Can you work these out from the drawing? Everything is in mm from the part's minimum corner. A direction names the side the tool comes from. Give positions to 0.01 mm unless a question says otherwise; leave off trailing zeros. Loops run counter-clockwise (first coordinate to the right, second up) from the corner with the lowest first, then second, coordinate; pieces in that order, holes last. Notation, with made-up numbers: (42.5, 42.5) - (98.5, 42.5) arc R23 cw to (98.5, 63.5) - close; hole circle Ø8 at (-34, -19). An arc over 180 degrees is marked (long way). Answer in a Markdown table with one row per item.
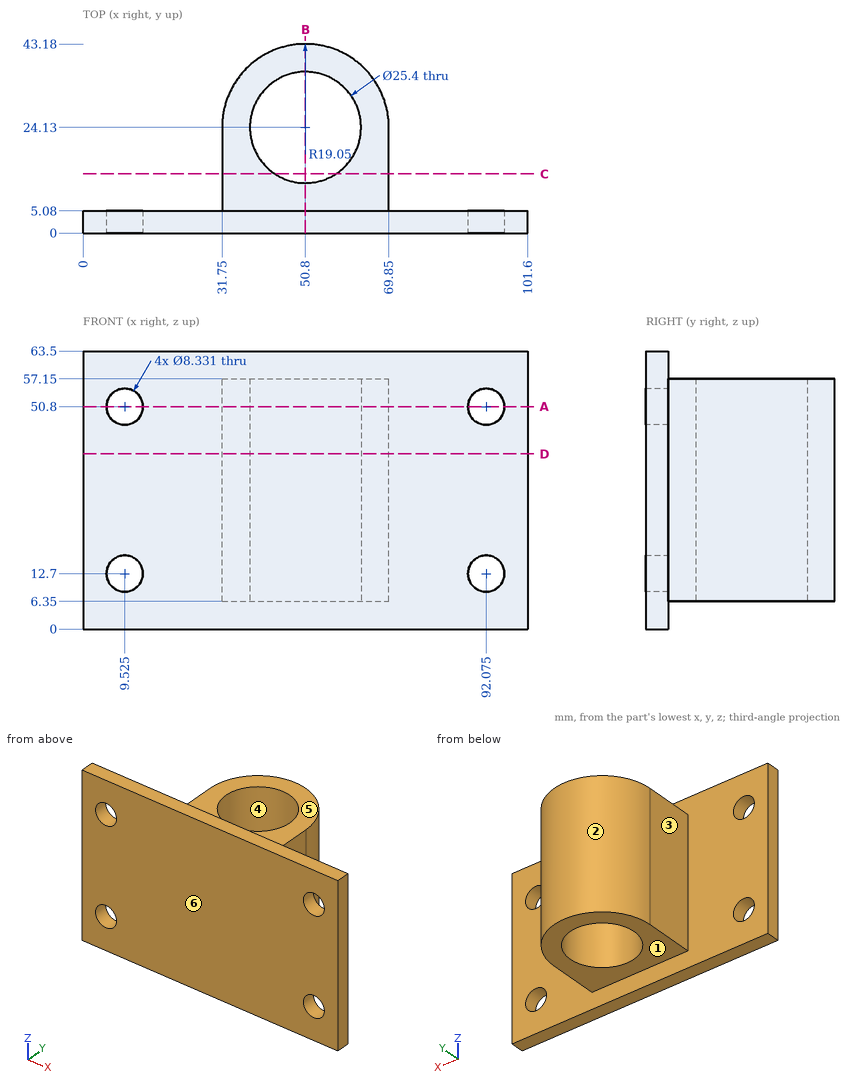
Q1. Imagine slicing it at C-C, the plane y = 13.5. Write out the boundary of the cut face in (x, z).
Checked values:
| item | result |
|---|---|
| outline | (31.75, 6.35) - (43.85, 6.35) - (43.85, 57.15) - (31.75, 57.15) - close; (57.75, 6.35) - (69.85, 6.35) - (69.85, 57.15) - (57.75, 57.15) - close |
Q2. If I drill on line 1 (X direction, y = 2.7, z = 12.7); line 2 (X direction, y = 23.5, z = 33); line 3 (X direction, y = 3, z = 50), over which ranges is the centre line in solid material (lowest first)? Write a range as [from, to].
Checked values:
| item | result |
|---|---|
| line 1 | x = [0, 5.36], [13.69, 87.91], [96.24, 101.6] |
| line 2 | x = [31.75, 38.12], [63.48, 69.85] |
| line 3 | x = [0, 5.44], [13.61, 87.99], [96.16, 101.6] |
Q3. Imagine slicing it at B-B, the plane x = 50.8. Write out the boundary of the cut face in (y, z).
Checked values:
| item | result |
|---|---|
| outline | (0, 0) - (5.08, 0) - (5.08, 6.35) - (11.43, 6.35) - (11.43, 57.15) - (5.08, 57.15) - (5.08, 63.5) - (0, 63.5) - close; (36.83, 6.35) - (43.18, 6.35) - (43.18, 57.15) - (36.83, 57.15) - close |
Q4. For pin 1 (5.5 mm diameter, centred on y = 14.5, z = 23.5, fed in from -X); pin 2 (10 mm diameter, centred on y = 13.5, z = 28, fed in from +X); pin 3 (1.5 mm diameter, centred on x = 68, y = 22, fed in from -Z); pin 4 (7.5 mm diameter, centred on x = 9.525, z = 50.8, fed in from -Y), each with a flat end and sliding along its axis, tell me the tip position at first contact or that it passes through.
Checked values:
| item | result |
|---|---|
| pin 1 | stops at x = 31.75 |
| pin 2 | stops at x = 69.85 |
| pin 3 | stops at z = 6.35 |
| pin 4 | passes through |
Q5. Imagine slicing it at D-D, the plane z = 40. Write out the boundary of the cut face in (x, y).
Checked values:
| item | result |
|---|---|
| outline | (0, 0) - (101.6, 0) - (101.6, 5.08) - (69.85, 5.08) - (69.85, 24.13) arc R19.05 ccw to (31.75, 24.13) - (31.75, 5.08) - (0, 5.08) - close; hole circle Ø25.4 at (50.8, 24.13) |
Q6. On a 3-axis mill with a long thin cutter (end or side, diameter ignored), from which of +Z, -Z, +X, -X, +Y, -Y can I reach the whole of each face in a straight line? I mean the marked faces 5 and 6. Say none if no direction works.
Checked values:
| item | result |
|---|---|
| face 5 | +Z, +X, -X, +Y |
| face 6 | +Z, -Z, +X, -X, -Y |
Q7. If we mould it in two halves opening along X, with no side actions, what happens to the marked faces 1, 2, 3 and 4? For each: released by +X, released by -X, zero draft, split by the parting line, or undercut.
Checked values:
| item | result |
|---|---|
| face 1 | zero draft |
| face 2 | split by the parting line |
| face 3 | released by -X |
| face 4 | undercut |
Q8. Imagine slicing it at A-A, the plane z = 50.8. Write out the boundary of the cut face in (x, y), and give its area (3 significant figures).
Checked values:
| item | result |
|---|---|
| outline | (0, 0) - (5.36, 0) - (5.36, 5.08) - (0, 5.08) - close; (13.69, 0) - (87.91, 0) - (87.91, 5.08) - (69.85, 5.08) - (69.85, 24.13) arc R19.05 ccw to (31.75, 24.13) - (31.75, 5.08) - (13.69, 5.08) - close; (96.24, 0) - (101.6, 0) - (101.6, 5.08) - (96.24, 5.08) - close; hole circle Ø25.4 at (50.8, 24.13) |
| area | 1,220 mm² |
